For this review, take the finished solid that the model builds, in its own axes (mm). Face numbers are marked on the shaded views. Give positions to 0.01 mm unless a question says otherwise; leave off trailing zeros. Order: outer loops, then holes, each group sorted by start corner. A loop starts at its lowest first (then second) coordinate and runs counter-clockwise, first axis right, second up. Notation, with made-up numbers: (18.5, -2.75) - (70.5, -2.75) arc R37 cw to (70.5, 34.25) - close; hole circle Ø2 at (-35, 81). An arc over 180 degrees is marked (long way). Use a Markdown table: item, result. Add a question column.
1) We need section B-B on y = -0.55. Write out the cut boundary in (x, z).
2) Clearance check with flat-ended pins moving along their axes: P1, Ø1.1, axis at x = 2.5, y = -0.5, coming from the -Z side; P2, Ø0.9, axis at x = 0, z = -5, coming from the -Y side; P3, Ø0.6, axis at y = 0, z = -2, coming from the -X side. State where each tip first meets the part, or that it passes through.
3) Wall thickness on L1, parallel to Z at x = 2.54, y = 1.2; L2, parallel to Y at x = 0.25, z = 5.75 (3 decimals); L3, parallel to Z at x = 1.75, y = -0.3: over which ranges is each line inside the solid? List them lowest first.
4) We need section C-C on z = 0.5. Write out the cut boundary in (x, y), then the cut area to 3 significant figures.
5) Mouldability with a two-part tool opening along X and no side actions: class the marked faces 1 and 2 as released by +X, released by -X, zero draft, split by the parting line, or undercut.
6) We need section D-D on z = 10.2. Write out the cut boundary in (x, y) (3 decimals).
7) We need section A-A on x = 2.54. Write out the cut boundary in (y, z) (3 decimals), then the cut area to 3 significant figures.
```python
from build123d import *

# Parameters (mm, degrees)
SKETCH005_W     = 7.4
SKETCH005_H     = 10.4
SKETCH005_R     = 1.58
PAD003_DEPTH    = 0.985
PAD001_DEPTH    = 4
POCKET_DEPTH    = 1.35
SKETCH004_R     = 1.6
POCKET001_DEPTH = 3.251
SKETCH006_R     = 2
POCKET002_DEPTH = 0.02
PAD_DEPTH       = 0.2625


with BuildPart() as pad003:
    # Sketch005 → Pad003 (new body, symmetric)
    with BuildSketch(Plane.XZ.offset(-1)):
        with Locations((2.54, 8.4)):
            Rectangle(SKETCH005_W, SKETCH005_H)
        with Locations((2.54, 10.2)):
            Circle(SKETCH005_R, mode=Mode.SUBTRACT)
    extrude(amount=PAD003_DEPTH, both=True)


with BuildPart() as pocket002:
    # Sketch001 → Pad001 (new body, symmetric)
    with BuildSketch(Plane.YZ.offset(2.54)):
        Polygon((0, 3), (-1.25, 3), (-1.25, 13.99), (-1.24, 14), (2, 14), (2, 3), align=None)
    extrude(amount=PAD001_DEPTH, both=True)

    # Sketch003 → Pocket (cut)
    with BuildSketch(Plane(origin=(2.54, -1.25, 0), x_dir=(0, 0, -1), z_dir=(0, -1, 0))):
        with BuildLine():
            Line((-12.219868, 0.5), (-12.219868, -0.5))
            Line((-12.219868, -0.5), (-11.719868, -0.5))
            ThreePointArc((-11.719868, -0.5), (-11, -1.385641), (-9.873078, -1.566245))
            Line((-9.623078, -1.999257), (-9.873078, -1.566245))
            Line((-8.757053, -1.499257), (-9.623078, -1.999257))
            Line((-9.007053, -1.066245), (-8.757053, -1.499257))
            ThreePointArc((-9.007053, -1.066245), (-8.6, 0), (-9.007053, 1.066245))
            Line((-8.757053, 1.499257), (-9.007053, 1.066245))
            Line((-9.623078, 1.999257), (-8.757053, 1.499257))
            Line((-9.873078, 1.566245), (-9.623078, 1.999257))
            ThreePointArc((-9.873078, 1.566245), (-11, 1.385641), (-11.719868, 0.5))
            Line((-12.219868, 0.5), (-11.719868, 0.5))
        make_face()
    extrude(amount=-POCKET_DEPTH, mode=Mode.SUBTRACT)

    # Sketch004 → Pocket001 (cut, through all)
    with BuildSketch(Plane(origin=(2.54, -1.25, 0), x_dir=(0, 0, -1), z_dir=(0, -1, 0))):
        with Locations((-10.2, 0)):
            Circle(SKETCH004_R)
    extrude(amount=-POCKET001_DEPTH, mode=Mode.SUBTRACT)

    # Sketch006 → Pocket002 (cut)
    with BuildSketch(Plane(origin=(2.54, 2, 0), x_dir=(0, 0, 1), z_dir=(0, 1, 0))):
        with BuildLine():
            Line((5.8, 3), (12.2, 3))
            ThreePointArc((13, 2.2), (12.765685, 2.765685), (12.2, 3))
            Line((13, 2.2), (13, -2.2))
            ThreePointArc((12.2, -3), (12.765685, -2.765685), (13, -2.2))
            Line((12.2, -3), (5.8, -3))
            ThreePointArc((5, -2.2), (5.234315, -2.765685), (5.8, -3))
            Line((5, -2.2), (5, 2.2))
            ThreePointArc((5.8, 3), (5.234315, 2.765685), (5, 2.2))
        make_face()
        with Locations((10.2, 0)):
            Circle(SKETCH006_R, mode=Mode.SUBTRACT)
    extrude(amount=-POCKET002_DEPTH, mode=Mode.SUBTRACT)


with BuildPart() as to_126_2_vertical:
    # Sketch → Pad (new body, symmetric)
    with BuildSketch(Plane.XZ):
        Polygon((-0.4, 0.3025), (-0.4, 0), (-0.4, -9.679469), (0, -9.75), (0.4, -9.679469), (0.4, 0), (0.4, 0.3025), (0.4, 3.73), (-0.4, 3.73), align=None)
        Polygon((4.68, 0.3025), (4.68, 0), (4.68, -9.679469), (5.08, -9.75), (5.48, -9.679469), (5.48, 0), (5.48, 0.3025), (5.48, 3.73), (4.68, 3.73), align=None)
    extrude(amount=PAD_DEPTH, both=True)

    add(pad003.part)
    add(pocket002.part)


solid = to_126_2_vertical.part
```
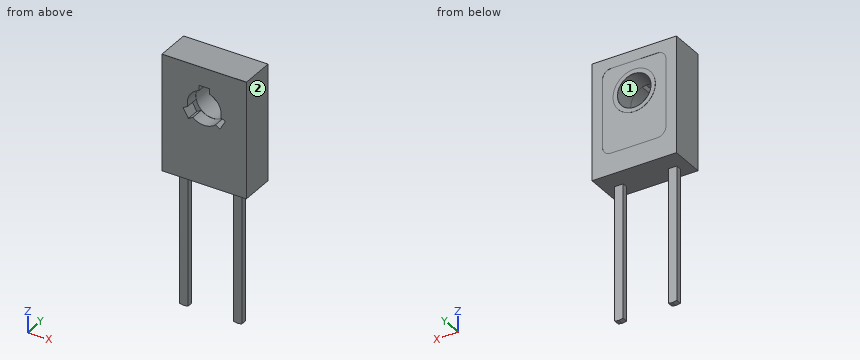
Checked values:
| question | item | result |
|---|---|---|
| 1 | outline | (-1.46, 3) - (6.54, 3) - (6.54, 14) - (-1.46, 14) - close; hole (0.54, 9.62) - (1.04, 8.76) - (1.47, 9.01) arc R1.6 ccw to (3.61, 9.01) - (4.04, 8.76) - (4.54, 9.62) - (4.11, 9.87) arc R1.6 ccw to (3.04, 11.72) - (3.04, 12.22) - (2.04, 12.22) - (2.04, 11.72) arc R1.6 ccw to (0.97, 9.87) - close |
| 2 | P1 | z = 3 |
| 2 | P2 | y = -0.26 |
| 2 | P3 | x = -0.4 |
| 3 | L1 | 3 to 8.62, 11.78 to 14 |
| 3 | L2 | -1.25 to 1.985 |
| 3 | L3 | 3 to 8.81, 11.59 to 14 |
| 4 | outline | (-0.4, -0.26) - (0.4, -0.26) - (0.4, 0.26) - (-0.4, 0.26) - close; (4.68, -0.26) - (5.48, -0.26) - (5.48, 0.26) - (4.68, 0.26) - close |
| 4 | area | 0.840 mm² |
| 5 | face 1 | undercut |
| 5 | face 2 | released by +X |
| 6 | outline | (-1.46, -1.25) - (0.94, -1.25) - (0.94, 0.015) - (0.96, 0.015) - (0.96, 1.985) - (0.94, 1.985) - (0.94, 2) - (0.54, 2) - (0.54, 1.985) - (-0.46, 1.985) - (-0.46, 2) - (-1.46, 2) - close; (4.12, 0.015) - (4.14, 0.015) - (4.14, -1.25) - (6.54, -1.25) - (6.54, 2) - (5.54, 2) - (5.54, 1.985) - (4.54, 1.985) - (4.54, 2) - (4.14, 2) - (4.14, 1.985) - (4.12, 1.985) - close |
| 7 | outline | (-1.25, 3) - (2, 3) - (2, 5) - (1.985, 5) - (1.985, 8.2) - (2, 8.2) - (2, 8.6) - (1.985, 8.6) - (1.985, 8.62) - (0.015, 8.62) - (0.015, 8.6) - (-1.25, 8.6) - close; (-1.25, 12.22) - (0.015, 12.22) - (0.015, 11.78) - (1.985, 11.78) - (1.985, 11.8) - (2, 11.8) - (2, 12.2) - (1.985, 12.2) - (1.985, 13) - (2, 13) - (2, 14) - (-1.24, 14) - (-1.25, 13.99) - close |
| 7 | area | 24.8 mm² |
